Build history of the part. All positions in model axes, mm. A direction names the side the tool comes from. Round coordinates to 2 decimals unless told otherwise and drop trailing zeros. Write each loop counter-clockwise with the first axis right and the second up, starting at its lowest first coordinate (ties: lowest second). Pieces come first, ordered by that corner, then holes.
Autodesk Inventor part; units mm, degrees
ref_plane "screw_XY" through (0, 5.6, 8) normal (0, 1, 0) x (1, 0, 0)
ref_plane "screw_YZ" through (0, 5.6, 8) normal (1, 0, 0) x (0, 0, -1)
ref_plane "screw_ZX" through (0, 5.6, 8) normal (0, 0, -1) x (0, 1, 0)
sketch "Sketch_1" plane through (0, 0, 0) normal (0, 0, 1) x (1, 0, 0)
  arc A0 (-4.95, 8.6889) -> (-4.95, -8.6889) centre (0, 0) ccw
  line L0 (-4.95, -8.6889) -> (-4.95, -22)
  line L1 (-4.95, -22) -> (4.95, -22)
  line L2 (4.95, -22) -> (4.95, -8.6889)
  arc A1 (4.95, -8.6889) -> (4.95, 8.6889) centre (0, 0) ccw
  line L3 (4.95, 8.6889) -> (4.95, 22)
  line L4 (4.95, 22) -> (-4.95, 22)
  line L5 (-4.95, 22) -> (-4.95, 8.6889)
extrude "Extrusion1" add sketch "Sketch_1" along normal blind 4.5
sketch "Sketch_2" plane through (0, 0, 0) normal (0, 1, 0) x (-1, 0, 0)
  circle A0 centre (0, 8) radius 5.5
extrude "Extrusion2" cut sketch "Sketch_2" along normal mid plane 44
sketch "Sketch_3" plane through (0, 0, 0) normal (0, 0, 1) x (1, 0, 0)
  arc A0 (-4.9135, 5.6) -> (-4.9135, -5.6) centre (0, 0) ccw
  line L0 (-4.9135, -5.6) -> (4.9135, -5.6)
  arc A1 (4.9135, -5.6) -> (4.9135, 5.6) centre (0, 0) ccw
  line L1 (4.9135, 5.6) -> (-4.9135, 5.6)
extrude "Extrusion3" add sketch "Sketch_3" along normal blind 16
sketch "Sketch_4" plane through (0, 0, 0) normal (0, 1, 0) x (-1, 0, 0)
  circle A0 centre (0, 8) radius 3.1
extrude "Extrusion4" cut sketch "Sketch_4" along normal mid plane 11.2
ref_plane "screw_XY" through (0, 5.6, 8) normal (0, 1, 0) x (1, 0, 0)
ref_plane "screw_YZ" through (0, 5.6, 8) normal (1, 0, 0) x (0, 0, -1)
ref_plane "screw_ZX" through (0, 5.6, 8) normal (0, 0, -1) x (0, 1, 0)
properties part number "HDJSN8-45__j"
1) Slice it at A-A (x = 0). Write the cut outline in (y, z).
Results:
outline: (-22, 0) - (22, 0) - (22, 2.5) - (5.6, 2.5) - (5.6, 4.9) - (-5.6, 4.9) - (-5.6, 2.5) - (-22, 2.5) - close; (-5.6, 11.1) - (5.6, 11.1) - (5.6, 16) - (-5.6, 16) - close
2) Slice it at D-D (z = 10.5). Write the cut outline in (x, y), plus the area to 3 significant figures.
Results:
outline: (-4.91, -5.6) - (-1.83, -5.6) - (-1.83, 5.6) - (-4.91, 5.6) arc R7.45 ccw to start; (1.83, -5.6) - (4.91, -5.6) arc R7.45 ccw to (4.91, 5.6) - (1.83, 5.6) - close
area: 108 mm2
3) Slice it at C-C (y = -2.5). Write the cut outline in (x, z), plus the area to 3 significant figures.
Results:
outline: (-9.68, 0) - (9.68, 0) - (9.68, 4.5) - (7.02, 4.5) - (7.02, 16) - (-7.02, 16) - (-7.02, 4.5) - (-9.68, 4.5) - close; hole circle Ø6.2 at (0, 8)
area: 218 mm2
4) Slice it at B-B (z = 8). Write the cut outline in (x, y), plus the area to 3 significant figures.
Results:
outline: (-4.91, -5.6) - (-3.1, -5.6) - (-3.1, 5.6) - (-4.91, 5.6) arc R7.45 ccw to start; (3.1, -5.6) - (4.91, -5.6) arc R7.45 ccw to (4.91, 5.6) - (3.1, 5.6) - close
area: 80.0 mm2
5) Mould opens along X. For faces 1 (the flat face through (-4.95, -15, 2)), 2 (the cylindrical face through (10, 0, 2)), 3 (the cylindrical face through (0.404, -0.078, 4.926)), 4 (the cylindrical face through (-0.1, 13.7, 2.5)) say: released by +X, released by -X, zero draft, split by the parting line, or undercut.
Results:
face 1: released by -X
face 2: released by +X
face 3: undercut
face 4: undercut
6) Which spindle directions (+Z, -Z, +X, -X, +Y, -Y) get a long thin tool onto all of the face, cutting with end or side? Do faces 5 (the flat face through (8, 0, 4.5)), 6 (the cylindrical face through (-0.1, -13.9, 2.5)), 7 (the flat face through (-8, 0, 4.5)), 8 (the flat face through (-4.95, 15, 2)). Say none if no direction does.
Results:
face 5: +Z, +X
face 6: +Z, -Y
face 7: +Z, -X
face 8: +Z, -Z, -X, +Y
7) Wall check: L1, parallel to Z at x = 0, y = -3; L2, parallel to Y at x = 4.25, z = 10.5; L3, parallel to Z at x = -6.25, y = 5.5. Give the ranges that are in metal, low to high.
Results:
L1: z = 0 to 4.9, 11.1 to 16
L2: y = -5.6 to 5.6
L3: z = 0 to 4.5
8) Pin check, flat tips, straight feed: pin 1 Ø5 at (y, z) = (-2.5, 11.5) entering from +X; pin 2 Ø6 at (x, y) = (3, -6.5) entering from -Z; pin 3 Ø3.5 at (y, z) = (17, 1.5) entering from -X; pin 4 Ø2 at (y, z) = (14.5, 3) entering from +X. Stop position of each tip, or through.
Results:
pin 1: stops at x = 7.45
pin 2: stops at z = 0
pin 3: stops at x = -4.95
pin 4: stops at x = 4.95
